```python
from build123d import *

# Parameters (mm, degrees)
F1_DEPTH = 2
F2_R     = 0.99999
F3_SIZE  = 0.2


# Not quite as in the source:
# - a fillet or chamfer is up to 0.001 mm smaller than in the source, because OpenCascade refuses the exact size


with BuildPart() as f1:
    # F0 (on Top) → F1 (new body)
    with BuildSketch(Plane.XY):
        Polygon((-0.75, 5), (-0.75, 0), (-0.75, -3.5), (-2.75, -3.5), (-2.75, -0.5), (-4.25, -0.5), (-4.25, -5), (0.75, -5), (0.75, 0), (0.75, 3.5), (2.75, 3.5), (2.75, 0.5), (4.25, 0.5), (4.25, 5), align=None)
    extrude(amount=F1_DEPTH)

    # F2 (radius 1 in the source; OpenCascade refuses exactly that, so slightly less here)
    f2_edges = [f1.edges().sort_by_distance(p)[0] for p in [
        (-0.75, 5, 1),
        (0.75, 3.5, 1),
        (2.75, 3.5, 1),
        (4.25, 5, 1),
        (4.25, 0.5, 1),
        (0.75, -5, 1),
        (-4.25, -5, 1),
        (-4.25, -0.5, 1),
        (-0.75, -3.5, 1),
        (-2.75, -3.5, 1),
    ]]
    fillet(f2_edges, radius=F2_R)

    # F3
    f3_edges = [f1.edges().sort_by_distance(p)[0] for p in [
        (-0.75, 0.75, 0),
        (-0.45711, 4.70711, 0),
        (-1.04289, -3.20711, 0),
        (1.75, 5, 0),
        (-1.75, -3.5, 0),
        (3.95711, 4.70711, 0),
        (-2.45711, -3.20711, 0),
        (4.25, 2.75, 0),
        (-2.75, -1.500005, 0),
        (3.95711, 0.79289, 0),
        (-3.000005, -0.5, 0),
        (3.000005, 0.5, 0),
        (-3.95711, -0.79289, 0),
        (2.75, 1.500005, 0),
        (-4.25, -2.75, 0),
        (2.45711, 3.20711, 0),
        (-3.95711, -4.70711, 0),
        (1.75, 3.5, 0),
        (-1.75, -5, 0),
        (1.04289, 3.20711, 0),
        (0.45711, -4.70711, 0),
        (0.75, -0.75, 0),
    ]]
    chamfer(f3_edges, length=F3_SIZE)


solid = f1.part
```
Check sheet for the modelled part. Datum: model origin and axes. Units: mm. A direction names the side the tool comes from. Give positions to 0.01 mm unless a question says otherwise; leave off trailing zeros. Order: outer loops, then holes, each group sorted by start corner. A loop starts at its lowest first (then second) coordinate and runs counter-clockwise, first axis right, second up. Notation, with made-up numbers: (-29, -10.75) -> (9, -10.75) arc R16 ccw to (9, 11.25) -> close; hole circle Ø2 at (-2.5, -17). An arc over 180 degrees is marked (long way). Use CSV: the item, a comma, the result in double quotes. Start each with the question number.
1) Material ranges on line 1 (X direction, y = 2, z = 0.9); line 2 (X direction, y = -2.25, z = 0.75); line 3 (Y direction, x = -3, z = 0.6), recorded low to high. Write a range as from..to.
2) Sectioned sample at A-A, the plane y = -2. Record the boundary of the cut face in (x, z), plus the area to 3 significant figures.
3) Set-up check for faces 1 (the face through (-0.75, 1, 1)), 2 (the face through (-3.949, -0.785, 1.113)), 3 (the face through (1.035, 3.199, 1.113)): record each of +Z, -Z, +X, -X, +Y, -Y from which the full face is reachable in a straight line by a thin tool's end or side.
4) Mould release check, pull along X, two halves, no side actions. Record for faces 4 (the face through (4.25, 3, 1)), 5 (the face through (0.75, -1, 1)), 6 (the face through (2, 5, 1)): released by +X, released by -X, zero draft, split by the parting line, or undercut.
5) Go/stop test with flat-tipped pins: P1, Ø1, axis at x = -2, y = -2.5, coming from the +Z side; P2, Ø1, axis at y = -3, z = 1.5, coming from the +X side. Record where each tip stops, or that it passes through.
Recorded:
1,line 1,"-0.75..0.75, 2.75..4.25"
1,line 2,"-4.25..-2.75, -0.75..0.75"
1,line 3,"-5..-0.5"
2,outline,"(-4.25, 0.2) -> (-4.05, 0) -> (-2.95, 0) -> (-2.75, 0.2) -> (-2.75, 2) -> (-4.25, 2) -> close; (-0.75, 0.2) -> (-0.55, 0) -> (0.55, 0) -> (0.75, 0.2) -> (0.75, 2) -> (-0.75, 2) -> close"
2,area,"5.92 mm2"
3,face 1,"+Z, -Z, +Y"
3,face 2,"+Z, -Z, -X, +Y"
3,face 3,"+Z, -Z, -Y"
4,face 4,"released by +X"
4,face 5,"undercut"
4,face 6,"zero draft"
5,P1,"through"
5,P2,"x = 0.75"
